Could you check a few things on this model? Use its own coordinates, in mm. Face numbers are marked on the shaded views. Coordinates: 2 decimals unless noted, no trailing zeros. Order: outer loops, then holes, each group sorted by start corner. A loop starts at its lowest first (then second) coordinate and runs counter-clockwise, first axis right, second up. Notation, with made-up numbers: (-4.5, 85.25) -> (35.5, 85.25) arc R21 cw to (35.5, 112.25) -> close; hole circle Ø4 at (53.5, -19.75). An arc over 180 degrees is marked (long way). Use a Markdown table: item, result. Add a question column.
1) Thinking about a two-plate mould opening in X: for the marked faces 1, 2 and 3, which applies, +X half, -X half, draft (parallel to the pull), parting line (faces both ways), or undercut?
2) If I drill on L1, parallel to Z at x = 0, y = 42; L2, parallel to Y at x = -10, z = -24, over which ranges is the centre line in solid material (lowest first)? Write a range as [from, to].
3) If we section it at B-B (x = 0): Write out the boundary of the cut face in (y, z), plus the area to 3 significant figures.
4) If we section it at A-A (z = 0): Write out the boundary of the cut face in (x, y).
5) If we section it at C-C (y = 36): Write out the boundary of the cut face in (x, z).
6) Will these pins go through, and if not, where does the flat tip stop? pin 1 Ø5 at (x, z) = (-12, 2) entering from +Y; pin 2 Ø3 at (y, z) = (22.5, 18.5) entering from +X; pin 3 Ø1 at (x, y) = (-16.5, 37.5) entering from -Z.
Autodesk Fusion 360 part; units mm, degrees
sketch "Sketch1" plane through (0, 0, 0) normal (0, 1, 0) x (1, 0, 0)
  circle A0 centre (0, 0) radius 30
  circle A1 centre (0, 0) radius 27
  dimension "d1" = 60
  dimension "d2" = 54
extrude "Extrude1" add sketch "Sketch1" along normal blind 70 makes body 1
extrude "Extrude2" add sketch "Sketch1" along normal blind 4 contours A1 bodies 1
copy_body "Body->Comp1" bodies 1 removing the originals makes body 2 in component "tubeToolHolder01"
component "tubeToolHolder01" placed x (1, 0, 0) y (0, 1, 0) z (0, 0, 1) at (0, 0, 0)
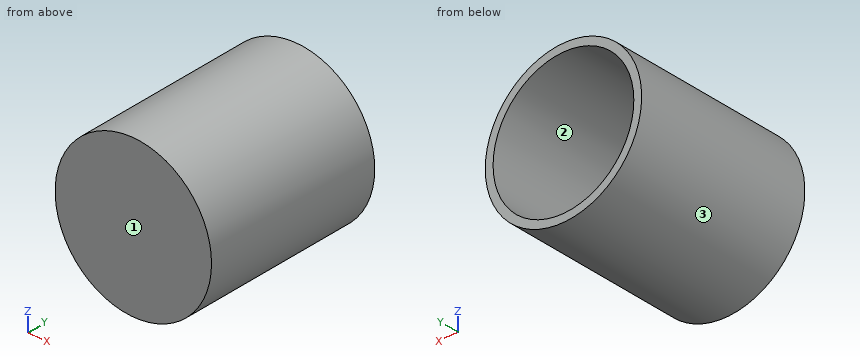
Answer sheet:
| question | item | result |
|---|---|---|
| 1 | face 1 | draft |
| 1 | face 2 | undercut |
| 1 | face 3 | parting line |
| 2 | L1 | [-30, -27], [27, 30] |
| 2 | L2 | [0, 4] |
| 3 | outline | (0, -30) -> (70, -30) -> (70, -27) -> (4, -27) -> (4, 27) -> (70, 27) -> (70, 30) -> (0, 30) -> close |
| 3 | area | 636 mm2 |
| 4 | outline | (-30, 0) -> (30, 0) -> (30, 70) -> (27, 70) -> (27, 4) -> (-27, 4) -> (-27, 70) -> (-30, 70) -> close |
| 5 | outline | circle Ø60 at (0, 0); hole circle Ø54 at (0, 0) |
| 6 | pin 1 | y = 4 |
| 6 | pin 2 | x = 24.72 |
| 6 | pin 3 | z = -25.38 |
